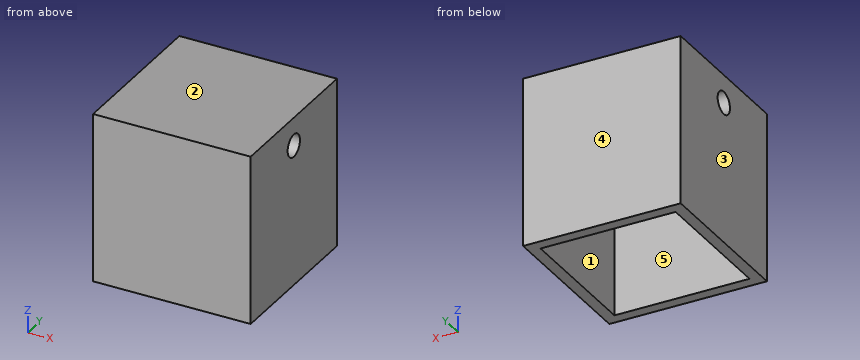
from build123d import *

# Parameters (mm, degrees)
SKETCH_1_W          = 14
SKETCH_1_H          = 14
SKETCH_1_W_2        = 12
SKETCH_1_H_2        = 12
EXTRUDE_1_DEPTH     = 10
SKETCH_2_W          = 14
SKETCH_2_H          = 14
EXTRUDE_2_DEPTH     = 5
SKETCH_3_R          = 1
CUT_EXTRUDE_1_DEPTH = 14


with BuildPart() as part:
    # 草图1 → 凸台-拉伸1 (new body)
    with BuildSketch(Plane.XY):
        with Locations((7, 7)):
            Rectangle(SKETCH_1_W, SKETCH_1_H)
        with Locations((7, 7)):
            Rectangle(SKETCH_1_W_2, SKETCH_1_H_2, mode=Mode.SUBTRACT)
    extrude(amount=EXTRUDE_1_DEPTH)

    # 草图2 → 凸台-拉伸2 (add)
    with BuildSketch(Plane.XY.offset(10)):
        with Locations((7, 7)):
            Rectangle(SKETCH_2_W, SKETCH_2_H)
    extrude(amount=EXTRUDE_2_DEPTH)

    # 草图3 → 切除-拉伸1 (cut)
    with BuildSketch(Plane(origin=(14, 0, 0), x_dir=(0, 0, -1), z_dir=(1, 0, 0))):
        with Locations((-12.5, 7)):
            Circle(SKETCH_3_R)
    extrude(amount=-CUT_EXTRUDE_1_DEPTH, mode=Mode.SUBTRACT)


solid = part.part
Can you work these out from the model? Positions are in its coordinate system, mm. Face numbers are marked on the shaded views. A direction names the side the tool comes from. Give positions to 0.01 mm unless a question says otherwise; leave off trailing zeros. Loops run counter-clockwise (first coordinate to the right, second up) from the corner with the lowest first, then second, coordinate; pieces in that order, holes last. Notation, with made-up numbers: M 77.25,-21 L 84.25,-21 A28 cw 84.25,13 Z; hole C 39,-17.75 d6. An arc over 180 degrees is marked long. One line per item, written item: value.
1) I'm going to push a flat-ended pin straight in: pin 1 (1.6 mm diameter, centred on y = 7, z = 12.5, fed in from -X). Where does the tip first touch, or does it pass through?
Geometry check:
pin 1: passes through
2) Thinking about a two-plate mould opening in X: for the marked faces 1, 2 and 3, which applies, +X half, -X half, draft (parallel to the pull), parting line (faces both ways), or undercut?
Geometry check:
face 1: undercut
face 2: draft
face 3: -X half
3) Imagine slicing it at B-B on x = 9. Write out the boundary of the cut face in (y, z), and give its area (3 significant figures).
Geometry check:
outline: M 0,0 L 1,0 L 1,10 L 13,10 L 13,0 L 14,0 L 14,15 L 0,15 Z; hole C 7,12.5 d2
area: 86.9 mm²
4) Imagine slicing it at C-C on z = 12.5. Write out the boundary of the cut face in (x, y).
Geometry check:
outline: M 0,0 L 14,0 L 14,6 L 0,6 Z; M 0,8 L 14,8 L 14,14 L 0,14 Z
5) Please list where these lines run through material, in increasing order: line 1 (X direction, y = 11, z = 8); line 2 (Y direction, x = 7.5, z = 12.5).
Geometry check:
line 1: x = 0 to 1, 13 to 14
line 2: y = 0 to 6, 8 to 14
6) Imagine slicing it at A-A on y = 7. Write out the boundary of the cut face in (x, z), and give its area (3 significant figures).
Geometry check:
outline: M 0,0 L 1,0 L 1,10 L 13,10 L 13,0 L 14,0 L 14,11.5 L 0,11.5 Z; M 0,13.5 L 14,13.5 L 14,15 L 0,15 Z
area: 62.0 mm²
7) On a 3-axis mill with a long thin cutter (end or side, diameter ignored), from which of +Z, -Z, +X, -X, +Y, -Y can I reach the whole of each face in a straight line? I mean the marked faces 4 and 5. Say none if no direction works.
Geometry check:
face 4: +Z, -Z, +X, -X, +Y
face 5: -Z
8) Imagine slicing it at D-D on z = 9.25. Write out the boundary of the cut face in (x, y), and give its area (3 significant figures).
Geometry check:
outline: M 0,0 L 14,0 L 14,14 L 0,14 Z; hole M 1,1 L 13,1 L 13,13 L 1,13 Z
area: 52.0 mm²
